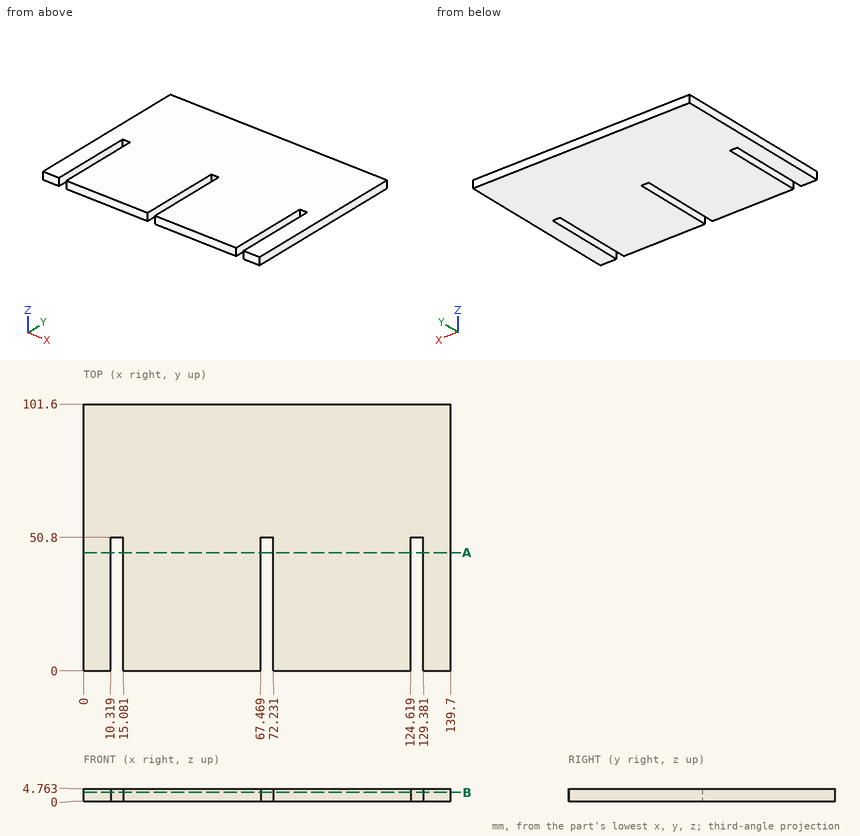
Check sheet for the drawn part. Datum: minimum x, y, z corner. Units: mm. Round coordinates to 2 decimals unless told otherwise and drop trailing zeros. Order: outer loops, then holes, each group sorted by start corner. A loop starts at its lowest first (then second) coordinate and runs counter-clockwise, first axis right, second up. Notation, with made-up numbers: M 60,-7.5 L 111,-7.5 A9 ccw 111,1.5 Z; hole C -18.5,-31.75 d4. An arc over 180 degrees is marked long. Answer in a Markdown table with one row per item.
(1) Section check A-A on y = 45. Record the boundary of the cut face in (x, z).
Findings:
| item | result |
|---|---|
| outline | M 0,0 L 10.32,0 L 10.32,4.76 L 0,4.76 Z; M 15.08,0 L 67.47,0 L 67.47,4.76 L 15.08,4.76 Z; M 72.23,0 L 124.62,0 L 124.62,4.76 L 72.23,4.76 Z; M 129.38,0 L 139.7,0 L 139.7,4.76 L 129.38,4.76 Z |
(2) Section check B-B on z = 3.45. Record the boundary of the cut face in (x, y).
Findings:
| item | result |
|---|---|
| outline | M 0,0 L 10.32,0 L 10.32,50.8 L 15.08,50.8 L 15.08,0 L 67.47,0 L 67.47,50.8 L 72.23,50.8 L 72.23,0 L 124.62,0 L 124.62,50.8 L 129.38,50.8 L 129.38,0 L 139.7,0 L 139.7,101.6 L 0,101.6 Z |
(3) Gauge pin test, flat ends, axial feed: pin 1 (2.5 mm diameter, centred on x = 13, z = 3, fed in from -Y); pin 2 (2.5 mm diameter, centred on y = 32, z = 1.5, fed in from -X). Record the tip position at first contact, or that the pin passes through.
Findings:
| item | result |
|---|---|
| pin 1 | stops at y = 50.8 |
| pin 2 | stops at x = 0 |
(4) Material ranges on line 1 along X through (y, z) = (25.5, 4); line 2 along Y through (x, z) = (69.5, 3.9), recorded low to high. Write a range as from..to.
Findings:
| item | result |
|---|---|
| line 1 | x = 0..10.32, 15.08..67.47, 72.23..124.62, 129.38..139.7 |
| line 2 | y = 50.8..101.6 |
